```python
from build123d import *

# Parameters (mm, degrees)
SKETCH1_W           = 90
SKETCH1_H           = 50
BOSS_EXTRUDE1_DEPTH = 30
SKETCH2_W           = 40.3
SKETCH2_H           = 40
CUT_EXTRUDE1_DEPTH  = 51
SKETCH3_R           = 4.1
CUT_EXTRUDE2_DEPTH  = 31
SKETCH4_R           = 8
CUT_EXTRUDE3_DEPTH  = 7


with BuildPart() as part:
    # Sketch1 → Boss-Extrude1 (new body)
    with BuildSketch(Plane(origin=(0, 0, 0), x_dir=(1, 0, 0), z_dir=(0, 1, 0))):
        Rectangle(SKETCH1_W, SKETCH1_H)
    extrude(amount=BOSS_EXTRUDE1_DEPTH)

    # Sketch2 → Cut-Extrude1 (cut, through all)
    with BuildSketch(Plane.XY.offset(25)):
        with Locations((0, 30)):
            Rectangle(SKETCH2_W, SKETCH2_H)
    extrude(amount=-CUT_EXTRUDE1_DEPTH, mode=Mode.SUBTRACT)

    # Sketch3 → Cut-Extrude2 (cut, through all)
    with BuildSketch(Plane.XZ):
        with Locations((-35, 15)):
            Circle(SKETCH3_R)
        with Locations((-35, -15)):
            Circle(SKETCH3_R)
        with Locations((35, -14.217273236)):
            Circle(SKETCH3_R)
        with Locations((35, 15)):
            Circle(SKETCH3_R)
    extrude(amount=-CUT_EXTRUDE2_DEPTH, mode=Mode.SUBTRACT)

    # Sketch4 → Cut-Extrude3 (cut)
    with BuildSketch(Plane.XZ):
        with Locations((35, 15)):
            Circle(SKETCH4_R)
        with Locations((35, -14.217273236)):
            Circle(SKETCH4_R)
        with Locations((-35, 15)):
            Circle(SKETCH4_R)
        with Locations((-35, -15)):
            Circle(SKETCH4_R)
    extrude(amount=-CUT_EXTRUDE3_DEPTH, mode=Mode.SUBTRACT)


solid = part.part
```
Geometry: final body of the model. Coordinates: model frame, mm. A direction names the side the tool comes from. Round coordinates to 2 decimals unless told otherwise and drop trailing zeros. Order: outer loops, then holes, each group sorted by start corner. A loop starts at its lowest first (then second) coordinate and runs counter-clockwise, first axis right, second up. Notation, with made-up numbers: M -29.5,-27 L -20.5,-27 A10 cw -20.5,-20 Z; hole C 23.5,-14.75 d5. An arc over 180 degrees is marked long. One line per item, written item: value.
(1) Pull-direction query (X, two-part tool) for faces 1 (the flat face through (32, 30, 0)), 2 (the cylindrical face through (-41.349, 3.451, -19.868)), 3 (the flat face through (45, 15, 0)), 4 (the cylindrical face through (31.746, 18.339, -16.712)); classes: pulls with the +X half, pulls with the -X half, needs draft (parallel to the pull), parting line crosses it, or undercut.
Result sheet:
face 1: needs draft
face 2: undercut
face 3: pulls with the +X half
face 4: undercut
(2) Line query: probe 1 along Z at (x, y) = (-35, 4); probe 2 along Z at (x, y) = (35, 20.5); probe 3 along X at (y, z) = (20.5, -6). Output: solid intervals per line, ascending. Write a range as [from, to].
Result sheet:
probe 1: [-25, -23], [-7, 7], [23, 25]
probe 2: [-25, -18.32], [-10.12, 10.9], [19.1, 25]
probe 3: [-45, -20.15], [20.15, 45]
(3) Cut plane D-D (z = 4). Return the cut outline in (x, y).
Result sheet:
outline: M -45,0 L 45,0 L 45,30 L 20.15,30 L 20.15,10 L -20.15,10 L -20.15,30 L -45,30 Z
(4) Cut plane C-C (x = -35). Return the cut outline in (y, z), and give its area (3 significant figures).
Result sheet:
outline: M 0,-25 L 30,-25 L 30,-19.1 L 7,-19.1 L 7,-23 L 0,-23 Z; M 0,-7 L 7,-7 L 7,-10.9 L 30,-10.9 L 30,10.9 L 7,10.9 L 7,7 L 0,7 Z; M 0,23 L 7,23 L 7,19.1 L 30,19.1 L 30,25 L 0,25 Z
area: 899 mm2
(5) Reachability of faces 5 (the flat face through (0, 10, 0)), 6 (the flat face through (-45, 15, 0)), 7 (the flat face through (31, 7, 17)) from +Z, -Z, +X, -X, +Y, -Y: full face, straight path, thin tool, end or side. Return the list, or none.
Result sheet:
face 5: +Z, -Z, +Y
face 6: +Z, -Z, -X, +Y, -Y
face 7: -Y
(6) Cut plane B-B (y = 28.25). Return the cut outline in (x, z), and give its area (3 significant figures).
Result sheet:
outline: M -45,-25 L -20.15,-25 L -20.15,25 L -45,25 Z; M 20.15,-25 L 45,-25 L 45,25 L 20.15,25 Z; hole C -35,-15 d8.2; hole C -35,15 d8.2; hole C 35,-14.22 d8.2; hole C 35,15 d8.2
area: 2,270 mm2
(7) Pin query (flat end, axial travel): P1, Ø6.5, axis at x = 35, z = 15, coming from the -Y side; P2, Ø13, axis at x = 34, z = 16, coming from the -Y side; P3, Ø20, axis at x = -6.5, z = 7.5, coming from the +Y side. Return the tip coordinate at first contact, or that it passes through.
Result sheet:
P1: through
P2: y = 7
P3: y = 10
(8) Cut plane A-A (z = 15). Return the cut outline in (x, y), and give its area (3 significant figures).
Result sheet:
outline: M -45,0 L -43,0 L -43,7 L -39.1,7 L -39.1,30 L -45,30 Z; M -30.9,7 L -27,7 L -27,0 L 27,0 L 27,7 L 30.9,7 L 30.9,30 L 20.15,30 L 20.15,10 L -20.15,10 L -20.15,30 L -30.9,30 Z; M 39.1,7 L 43,7 L 43,0 L 45,0 L 45,30 L 39.1,30 Z
area: 1,290 mm2
